```python
from build123d import *

# Parameters (mm, degrees)
BOSS_EXTRUDE1_DEPTH = 10
SKETCH9_R           = 2
CUT_EXTRUDE14_DEPTH = 181
SKETCH2_W           = 124
SKETCH2_H           = 124
CUT_EXTRUDE15_DEPTH = 6
SKETCH10_W          = 20
SKETCH10_H          = 31
CUT_EXTRUDE17_DEPTH = 2
SKETCH11_W          = 92
SKETCH11_H          = 95
CUT_EXTRUDE18_DEPTH = 1
FILLET3_R           = 11
SKETCH13_W          = 34.982721691
SKETCH13_H          = 0.5
BOSS_EXTRUDE3_DEPTH = 41


with BuildPart() as part:
    # Sketch1 → Boss-Extrude1 (new body)
    with BuildSketch(Plane(origin=(0, 0, 0), x_dir=(1, 0, 0), z_dir=(0, 1, 0))):
        Polygon((-67, -15), (-67, -67), (67, -67), (67, -15), (82, -15), (82, 15), (67, 15), (67, 67), (-67, 67), (-67, 15), (-82, 15), (-82, -15), align=None)
    extrude(amount=BOSS_EXTRUDE1_DEPTH)

    # Sketch9 → Cut-Extrude14 (cut)
    with BuildSketch(Plane(origin=(82, 0, 0), x_dir=(0, 0, -1), z_dir=(1, 0, 0))):
        with Locations((0, 3)):
            Circle(SKETCH9_R)
    extrude(amount=-CUT_EXTRUDE14_DEPTH, mode=Mode.SUBTRACT)

    # Sketch2 → Cut-Extrude15 (cut)
    with BuildSketch(Plane(origin=(0, 10, 0), x_dir=(1, 0, 0), z_dir=(0, 1, 0))):
        Rectangle(SKETCH2_W, SKETCH2_H)
    extrude(amount=-CUT_EXTRUDE15_DEPTH, mode=Mode.SUBTRACT)

    # Sketch10 → Cut-Extrude17 (cut)
    with BuildSketch(Plane(origin=(0, 4, 0), x_dir=(1, 0, 0), z_dir=(0, 1, 0))):
        with Locations((35.5, 0)):
            Rectangle(SKETCH10_W, SKETCH10_H)
        with Locations((-35.5, 0)):
            Rectangle(SKETCH10_W, SKETCH10_H)
    extrude(amount=-CUT_EXTRUDE17_DEPTH, mode=Mode.SUBTRACT)

    # Sketch11 → Cut-Extrude18 (cut)
    with BuildSketch(Plane(origin=(0, 4, 0), x_dir=(1, 0, 0), z_dir=(0, 1, 0))):
        Rectangle(SKETCH11_W, SKETCH11_H)
    extrude(amount=-CUT_EXTRUDE18_DEPTH, mode=Mode.SUBTRACT)

    # Fillet3
    fillet3_edges = [part.edges().sort_by_distance(p)[0] for p in [
        (62, 7, -62),
        (-62, 7, 62),
        (62, 7, 62),
        (-62, 7, -62),
    ]]
    fillet(fillet3_edges, radius=FILLET3_R)

    # Sketch13 → Boss-Extrude3 (add)
    with BuildSketch(Plane(origin=(0, 0, -67), x_dir=(-1, 0, 0), z_dir=(0, 0, -1))):
        with Locations((-49.508639155, 0.25)):
            Rectangle(SKETCH13_W, SKETCH13_H)
    extrude(amount=BOSS_EXTRUDE3_DEPTH)


solid = part.part
```
Input: part model. Units: mm. Frame: model coordinates. A direction names the side the tool comes from. Give positions to 0.01 mm unless a question says otherwise; leave off trailing zeros. Order: outer loops, then holes, each group sorted by start corner. A loop starts at its lowest first (then second) coordinate and runs counter-clockwise, first axis right, second up. Notation, with made-up numbers: (67, 44.25) - (110, 44.25) arc R10 cw to (110, 58.25) - close; hole circle Ø9 at (81.5, 75). An arc over 180 degrees is marked (long way). One line per item, written item: value.
1. Cut plane B-B, the plane x = -29.5. Output: boundary loops of the cut face in (y, z), and give its area (3 significant figures).
Determined:
outline: (0, -67) - (10, -67) - (10, -62) - (4, -62) - (4, -47.5) - (3, -47.5) - (3, -15.5) - (2, -15.5) - (2, -1.73) arc R2 cw to (2, 1.73) - (2, 15.5) - (3, 15.5) - (3, 47.5) - (4, 47.5) - (4, 62) - (10, 62) - (10, 67) - (0, 67) - close
area: 468 mm2
2. Draft query along Z for faces 6 (the face through (-1, 7, 62)), 7 (the face through (67, 5, -40)), 8 (the face through (75, 5, -15)). Return one class per face: released by +Z, released by -Z, zero draft, split by the parting line, or undercut.
Determined:
face 6: undercut
face 7: zero draft
face 8: released by -Z
3. Pin query (flat end, axial travel): pin 1 Ø4 at (x, z) = (-31.5, 7) entering from +Y; pin 2 Ø1.1 at (x, y) = (-40, 2.5) entering from -Z; pin 3 Ø3 at (y, z) = (4, -51) entering from -X. Return the tip coordinate at first contact, or that it passes through.
Determined:
pin 1: y = 2
pin 2: z = -67
pin 3: x = -67
4. Cut plane A-A, the plane y = 8.25. Output: boundary loops of the cut face in (x, z).
Determined:
outline: (-82, -15) - (-67, -15) - (-67, -67) - (67, -67) - (67, -15) - (82, -15) - (82, 15) - (67, 15) - (67, 67) - (-67, 67) - (-67, 15) - (-82, 15) - close; hole (-62, -51) arc R11 ccw to (-51, -62) - (51, -62) arc R11 ccw to (62, -51) - (62, 51) arc R11 ccw to (51, 62) - (-51, 62) arc R11 ccw to (-62, 51) - close
5. Line query: probe 1 along X at (y, z) = (5, 28); probe 2 along X at (y, z) = (8.75, -1). Output: solid intervals per line, ascending.
Determined:
probe 1: -67 to -62, 62 to 67
probe 2: -82 to -62, 62 to 82
6. Cut plane C-C, the plane z = -12.5. Output: boundary loops of the cut face in (x, y).
Determined:
outline: (-82, 0) - (82, 0) - (82, 10) - (62, 10) - (62, 4) - (46, 4) - (46, 3) - (45.5, 3) - (45.5, 2) - (25.5, 2) - (25.5, 3) - (-25.5, 3) - (-25.5, 2) - (-45.5, 2) - (-45.5, 3) - (-46, 3) - (-46, 4) - (-62, 4) - (-62, 10) - (-82, 10) - close
7. Cut plane D-D, the plane x = 11. Output: boundary loops of the cut face in (y, z).
Determined:
outline: (0, -67) - (10, -67) - (10, -62) - (4, -62) - (4, -47.5) - (3, -47.5) - (3, -2) arc R2 cw to (3, 2) - (3, 47.5) - (4, 47.5) - (4, 62) - (10, 62) - (10, 67) - (0, 67) - close
8. Reachability of faces 1 (the face through (-1, 7, -62)), 2 (the face through (-75, 5, 15)), 3 (the face through (-82, 6, 0)), 4 (the face through (-67, 5, -41)), 5 (the face through (74, 5, 15)) from +Z, -Z, +X, -X, +Y, -Y: full face, straight path, thin tool, end or side. Return the list, or none.
Determined:
face 1: +Y
face 2: +Z, -X, +Y, -Y
face 3: +Z, -Z, -X, +Y, -Y
face 4: -Z, -X, +Y, -Y
face 5: +Z, +X, +Y, -Y
